Source: CAD feature listing. Evaluate the final solid. Frame: model axes, mm. Coordinates: 2 decimals unless noted, no trailing zeros. Loops run counter-clockwise (first coordinate to the right, second up) from the corner with the lowest first, then second, coordinate; pieces in that order, holes last.
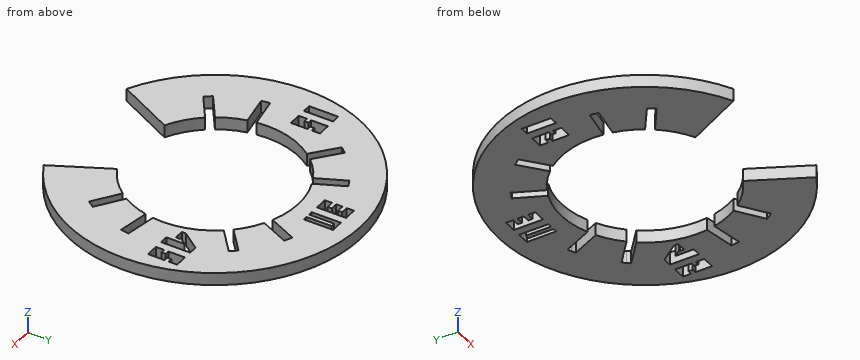
from build123d import *

# Parameters (mm, degrees)
BOSS_EXTRUDE1_DEPTH = 1.5
SKETCH2_W           = 1
SKETCH2_H           = 3.5
CUT_EXTRUDE1_DEPTH  = 1.5


with BuildPart() as part:
    # Sketch1 → Boss-Extrude1 (new body)
    with BuildSketch(Plane.XY):
        with BuildLine():
            Line((-4.539904997, -8.910065242), (-7.944833745, -15.592614173))
            ThreePointArc((-7.944833745, -15.592614173), (0, 17.5), (7.944833745, -15.592614173))
            Line((7.944833745, -15.592614173), (4.539904997, -8.910065242))
            ThreePointArc((4.539904997, -8.910065242), (0, 10), (-4.539904997, -8.910065242))
        make_face()
    extrude(amount=BOSS_EXTRUDE1_DEPTH)

    # Sketch2 → Cut-Extrude1 (cut)
    with BuildSketch(Plane.XY.offset(1.5)):
        with Locations((-14.718025133, 3.507588082)):
            Rectangle(SKETCH2_W, SKETCH2_H)
        Polygon((-13.218025133, 5.257588082), (-13.218025133, 3.257588082), (-12.718025133, 3.257588082), (-12.718025133, 2.757588082), (-13.218025133, 2.757588082), (-13.218025133, 1.757588082), (-11.718025133, 1.757588082), (-11.718025133, 3.757588082), (-12.218025133, 3.757588082), (-12.218025133, 4.257588082), (-11.718025133, 4.257588082), (-11.718025133, 5.257588082), align=None)
        Polygon((-2, 15.418453076), (-0.5, 15.418453076), (-0.5, 11.918453076), (-2, 11.918453076), (-2, 12.793453076), (-1.1452971, 12.793453076), (-1.1452971, 13.293453076), (-2, 13.293453076), (-2, 14.043453076), (-1.1452971, 14.043453076), (-1.1452971, 14.543453076), (-2, 14.543453076), align=None)
        Polygon((0.5, 15.418453076), (0.5, 11.918453076), (1, 11.918453076), (1, 12.418453076), (1, 14.918453076), (1.5, 14.918453076), (1.5, 12.418453076), (1.5, 11.918453076), (2, 11.918453076), (2, 15.418453076), align=None)
        Polygon((12.097744761, 5.231352171), (13.110444891, 5.231352171), (13.110444891, 1.731375213), (12.110444891, 1.731375213), (12.110444891, 3.922086384), (11.470557234, 3.073526548), (11.610444891, 3.073526548), (11.610444891, 2.572345702), (10.470557234, 2.572345702), (10.470557234, 3.073526548), align=None)
        Polygon((14.110444891, 5.231352171), (14.110444891, 3.231375213), (14.610444891, 3.231375213), (14.610444891, 2.731375213), (14.110444891, 2.731375213), (14.110444891, 1.731375213), (15.610444891, 1.731375213), (15.610444891, 3.731375213), (15.110444891, 3.731375213), (15.110444891, 4.231375213), (15.610444891, 4.231375213), (15.610444891, 5.231352171), align=None)
        Polygon((-11.232578871, -7.865136399), (-11.519367089, -7.455560377), (-8.468062853, -5.319014149), (-7.473400559, -4.622544113), (-6.899824123, -5.441696158), (-7.894486417, -6.138166194), (-10.945790653, -8.274712421), align=None)
        Polygon((-13.504123972, -2.381141407), (-13.590948061, -1.888737531), (-9.922583819, -1.24190594), (-8.726772681, -1.031052172), (-8.553124503, -2.015859925), (-9.748935641, -2.226713693), (-13.417299884, -2.873545284), align=None)
        Polygon((-10.504343712, 8.814190935), (-10.182949908, 9.197213156), (-7.329469079, 6.802858445), (-6.399293139, 6.022348157), (-7.042080748, 5.256303714), (-7.972256688, 6.036814002), (-10.825737517, 8.431168713), align=None)
        Polygon((-5.795130453, 12.427697361), (-5.341976559, 12.639006492), (-3.76774269, 9.263051065), (-3.254574893, 8.162559174), (-4.16088268, 7.739940912), (-4.674050477, 8.840432803), (-6.248284346, 12.21638823), align=None)
        Polygon((5.795130453, 12.427697361), (6.248284346, 12.21638823), (4.674050477, 8.840432803), (4.16088268, 7.739940912), (3.254574893, 8.162559174), (3.76774269, 9.263051065), (5.341976559, 12.639006492), align=None)
        Polygon((10.504343712, 8.814190935), (10.825737517, 8.431168713), (7.972256688, 6.036814002), (7.042080748, 5.256303714), (6.399293139, 6.022348157), (7.329469079, 6.802858445), (10.182949908, 9.197213156), align=None)
        Polygon((13.504123972, -2.381141407), (13.417299884, -2.873545284), (9.748935641, -2.226713693), (8.553124503, -2.015859925), (8.726772681, -1.031052172), (9.922583819, -1.24190594), (13.590948061, -1.888737531), align=None)
        Polygon((11.232578871, -7.865136399), (10.945790653, -8.274712421), (7.894486417, -6.138166194), (6.899824123, -5.441696158), (7.473400559, -4.622544113), (8.468062853, -5.319014149), (11.519367089, -7.455560377), align=None)
    extrude(amount=-CUT_EXTRUDE1_DEPTH, mode=Mode.SUBTRACT)


solid = part.part
Q1. Section D-D, the plane x = 0. Return the cut outline in (y, z).
Q2. Section B-B, the plane y = 8. Return the cut outline in (x, z).
Q3. Line query: line 1 along X through (y, z) = (14, 0.1); line 2 along Y through (x, z) = (-5, 0.2); line 3 along Y through (x, z) = (6, 0.7). Output: solid intervals per line, ascending.
Q4. Contact query for a flat-ended pin moving along its axis: pin 1 Ø0.8 at (y, z) = (2.5, 0.5) entering from +X. Output: stop coordinate, or through.
Q5. Section A-A, the plane y = 0. Return the cut outline in (x, z).
Q6. Section C-C, the plane z = 0.4. Count the separate pieces of the cut face and the enclosed holes in it, plus the area to 3 significant figures.
Derived:
1. outline: (10, 0) - (17.5, 0) - (17.5, 1.5) - (10, 1.5) - close
2. outline: (-15.56, 0) - (-10.31, 0) - (-10.31, 1.5) - (-15.56, 1.5) - close; (-8.76, 0) - (-6, 0) - (-6, 1.5) - (-8.76, 1.5) - close; (6, 0) - (8.76, 0) - (8.76, 1.5) - (6, 1.5) - close; (10.31, 0) - (15.56, 0) - (15.56, 1.5) - (10.31, 1.5) - close
3. line 1: x = -10.5 to -2, -0.5 to 0.5, 1 to 1.5, 2 to 10.5
3. line 2: y = -9.81 to -8.66, 8.66 to 9.54, 11.91 to 16.77
3. line 3: y = -11.78 to -8, 8 to 11.68, 12.33 to 16.44
4. pin 1: stops at x = 17.37
5. outline: (-17.5, 0) - (-10, 0) - (-10, 1.5) - (-17.5, 1.5) - close; (10, 0) - (17.5, 0) - (17.5, 1.5) - (10, 1.5) - close
6. separate pieces: 1
6. enclosed holes: 6
6. area: 494 mm2
